```python
from build123d import *

# Parameters (mm, degrees)
F0_W     = 7.62
F0_H     = 3.175
F1_DEPTH = 50.8
F0_H_2   = 9.8044
F0_W_2   = 4.6228
F0_H_3   = 4.6228
F2_DEPTH = 3.175
F3_W     = 7.62
F3_H     = 3.175
F4_DEPTH = 9.8044
F6_DEPTH = 25.4
F8_DEPTH = 25.4


with BuildPart() as f1:
    # F0 (on Front) → F1 (new body)
    with BuildSketch(Plane.XZ):
        with Locations((0, 6.4897)):
            Rectangle(F0_W, F0_H)
    extrude(amount=F1_DEPTH)

    # F0 (on Front) → F2 (join)
    with BuildSketch(Plane.XZ):
        Rectangle(F0_W, F0_H_2)
        Rectangle(F0_W_2, F0_H_3, mode=Mode.SUBTRACT)
    extrude(amount=F2_DEPTH)

    # F3 (on face) → F4 (join)
    with BuildSketch(Plane(origin=(0, 0, 4.9022), x_dir=(1, 0, 0), z_dir=(0, 0, -1))):
        with Locations((0, 49.2125)):
            Rectangle(F3_W, F3_H)
    extrude(amount=F4_DEPTH)

    # F5 (on face) → F6 (cut)
    with BuildSketch(Plane.XZ.offset(50.8)):
        Polygon((2.3114, -2.032073), (2.3114, 1.5875), (2.3114, 2.590727), (-2.3114, 2.590727), (-2.3114, -2.032073), align=None)
    extrude(amount=-F6_DEPTH, mode=Mode.SUBTRACT)

    # F7 (on face) → F8 (cut)
    with BuildSketch(Plane.XY.offset(8.0772)):
        Polygon((2.3114, -9.1948), (0, -9.1948), (-2.3114, -9.1948), (-2.3114, -13.8176), (2.3114, -13.8176), align=None)
    extrude(amount=-F8_DEPTH, mode=Mode.SUBTRACT)


solid = f1.part
```
Design review of the part built by this model. Coordinates are the model's own, in mm. A direction names the side the tool comes from. Give positions to 0.01 mm unless a question says otherwise; leave off trailing zeros. Order: outer loops, then holes, each group sorted by start corner. A loop starts at its lowest first (then second) coordinate and runs counter-clockwise, first axis right, second up. Notation, with made-up numbers: (58.25, -17) -> (113.25, -17) arc R33 cw to (113.25, 13) -> close; hole circle Ø4 at (73.25, 15). An arc over 180 degrees is marked (long way). Write each question's results on one line, items separated by ' | '. Start each with the question number.
Q1. Machinability: for faces 4 (the flat face through (0, -9.195, 7)), 5 (the flat face through (0, -25, 4.902)), 6 (the flat face through (0, -2, -2.311)), which of the approach directions +Z, -Z, +X, -X, +Y, -Y give a long, thin tool a straight path to every point of the face, cutting with its end or side? Answer none if there is none.
Q2. Add section A-A on z = 4.25. Give the boundary of the cut face in (x, y) (3 decimals).
Q3. Add section D-D on x = -0.25. Give the boundary of the cut face in (y, z) (3 decimals).
Q4. Add section B-B on z = 1.5. Give the boundary of the cut face in (x, y) (3 decimals).
Q5. Mouldability with a two-part tool opening along Y and no side actions: class faces 1 (the flat face through (0, -50.8, 3)), 2 (the flat face through (0, -49, -4.902)), 3 (the flat face through (2.311, -12, 7)) as +Y half, -Y half, draft (parallel to the pull), parting line (faces both ways), or undercut.
Q6. Wall thickness on L1, parallel to Y at x = 2.75, z = 1.5 (3 decimals); L2, parallel to X at y = -13.5, z = 5.75; L3, parallel to Y at x = 1.75, z = 5.5: over which ranges is each line inside the solid? List them lowest first. Write a range as from..to.
Q7. Add section C-C on y = -10.5. Give the boundary of the cut face in (x, z).
Q8. For pin 1 (2.5 mm diameter, centred on x = 0.5, y = -16, fed in from -Z), flat-tipped, find the tip position at first contact; note if it passes through.
Found:
1) face 4: +Z, -Z | face 5: -Z, +X, -X | face 6: +Y
2) outline: (-3.81, -50.8) -> (3.81, -50.8) -> (3.81, -47.625) -> (-3.81, -47.625) -> close; (-3.81, -3.175) -> (3.81, -3.175) -> (3.81, 0) -> (-3.81, 0) -> close
3) outline: (-50.8, -4.902) -> (-47.625, -4.902) -> (-47.625, -2.032) -> (-50.8, -2.032) -> close; (-50.8, 2.591) -> (-47.625, 2.591) -> (-47.625, 4.902) -> (-13.818, 4.902) -> (-13.818, 8.077) -> (-50.8, 8.077) -> close; (-9.195, 4.902) -> (-3.175, 4.902) -> (-3.175, 2.311) -> (0, 2.311) -> (0, 8.077) -> (-9.195, 8.077) -> close; (-3.175, -4.902) -> (0, -4.902) -> (0, -2.311) -> (-3.175, -2.311) -> close
4) outline: (-3.81, -50.8) -> (-2.311, -50.8) -> (-2.311, -47.625) -> (-3.81, -47.625) -> close; (-3.81, -3.175) -> (-2.311, -3.175) -> (-2.311, 0) -> (-3.81, 0) -> close; (2.311, -50.8) -> (3.81, -50.8) -> (3.81, -47.625) -> (2.311, -47.625) -> close; (2.311, -3.175) -> (3.81, -3.175) -> (3.81, 0) -> (2.311, 0) -> close
5) face 1: -Y half | face 2: draft | face 3: undercut
6) L1: y = -50.8..-47.625, -3.175..0 | L2: x = -3.81..-2.31, 2.31..3.81 | L3: y = -50.8..-13.82, -9.19..0
7) outline: (-3.81, 4.9) -> (-2.31, 4.9) -> (-2.31, 8.08) -> (-3.81, 8.08) -> close; (2.31, 4.9) -> (3.81, 4.9) -> (3.81, 8.08) -> (2.31, 8.08) -> close
8) pin 1: stops at z = 4.9
